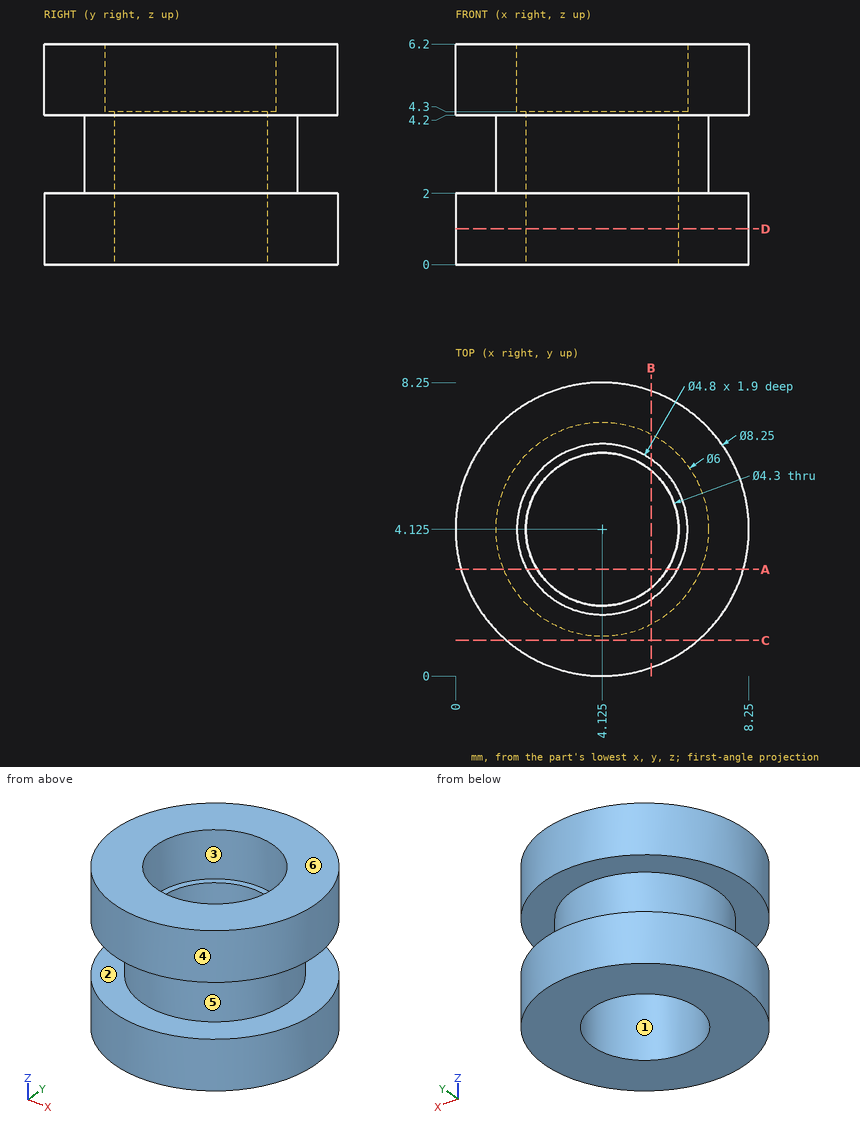
Can you work these out from the drawing? Everything is in mm from the part's minimum corner. A direction names the side the tool comes from. Round coordinates to 2 decimals unless told otherwise and drop trailing zeros. Write each loop counter-clockwise with the first axis right and the second up, starting at its lowest first coordinate (ties: lowest second). Pieces come first, ordered by that corner, then holes.
1. For the marked faces 1, 2 and 3, which set-ups out of +Z, -Z, +X, -X, +Y, -Y let a thin tool reach every point of the face, with its end or its side?
2. Suppose I cut it at B-B (x = 5.5). List the corners of the cut face in (y, z) for me, and give its area (3 significant figures).
3. Suppose I cut it at A-A (y = 3). List the corners of the cut face in (x, z) for me (3 decimals).
4. If we mould it in two halves opening along Z, with no side actions, what happens to the marked faces 4, 5 and 6? For each: released by +Z, released by -Z, zero draft, split by the parting line, or undercut.
5. Suppose I cut it at D-D (z = 1). List the corners of the cut face in (x, y) for me (3 decimals).
6. Will these pins go through, and if not, where does the flat tip stop? pin 1 Ø1.5 at (y, z) = (7.5, 2.5) entering from -X; pin 2 Ø1 at (x, z) = (7, 4) entering from +Y; pin 3 Ø2.5 at (x, y) = (3.5, 6) entering from +Z.
7. Suppose I cut it at C-C (y = 1). List the corners of the cut face in (x, z) for me.
8. I need wall thicknesses on L1, parallel to Z at x = 7, y = 1.5; L2, parallel to Y at x = 6, z = 5.5; L3, parallel to X at y = 4, z = 6. Which ranges of each line are inside material? Lowest first, please.
Answer sheet:
1. face 1: +Z, -Z
1. face 2: none
1. face 3: +Z
2. outline: (0.24, 0) - (2.47, 0) - (2.47, 4.3) - (2.16, 4.3) - (2.16, 6.2) - (0.24, 6.2) - (0.24, 4.2) - (1.46, 4.2) - (1.46, 2) - (0.24, 2) - close; (5.78, 0) - (8.01, 0) - (8.01, 2) - (6.79, 2) - (6.79, 4.2) - (8.01, 4.2) - (8.01, 6.2) - (6.09, 6.2) - (6.09, 4.3) - (5.78, 4.3) - close
2. area: 21.2 mm2
3. outline: (0.156, 0) - (2.293, 0) - (2.293, 4.3) - (2.005, 4.3) - (2.005, 6.2) - (0.156, 6.2) - (0.156, 4.2) - (1.344, 4.2) - (1.344, 2) - (0.156, 2) - close; (5.957, 0) - (8.094, 0) - (8.094, 2) - (6.906, 2) - (6.906, 4.2) - (8.094, 4.2) - (8.094, 6.2) - (6.245, 6.2) - (6.245, 4.3) - (5.957, 4.3) - close
4. face 4: zero draft
4. face 5: undercut
4. face 6: released by +Z
5. outline: circle Ø8.25 at (4.125, 4.125); hole circle Ø4.3 at (4.125, 4.125)
6. pin 1: stops at x = 1.11
6. pin 2: stops at y = 7.47
6. pin 3: stops at z = 6.2
7. outline: (1.43, 0) - (6.82, 0) - (6.82, 2) - (1.43, 2) - close; (1.43, 4.2) - (6.82, 4.2) - (6.82, 6.2) - (1.43, 6.2) - close
8. L1: z = 0 to 2, 4.2 to 6.2
8. L2: y = 0.45 to 2.63, 5.62 to 7.8
8. L3: x = 0 to 1.73, 6.52 to 8.25
